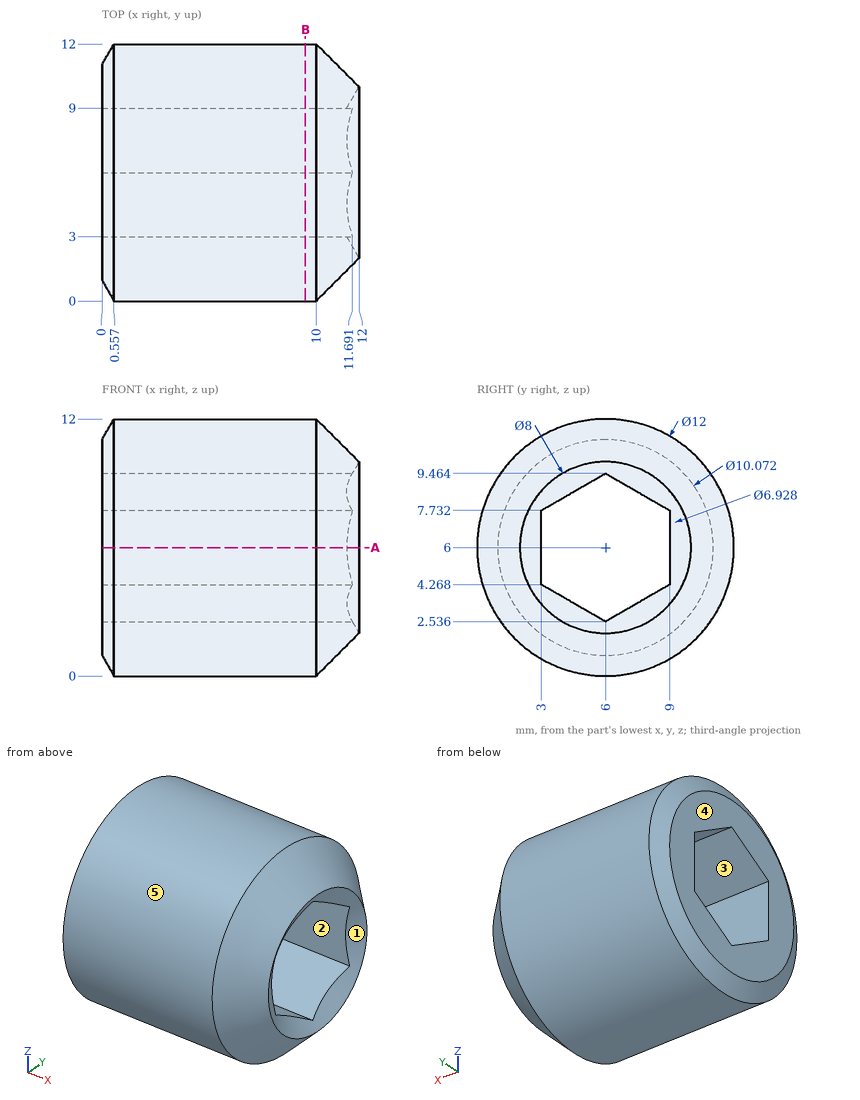
Can you work these out from the drawing? Everything is in mm from the part's minimum corner. A direction names the side the tool comes from. Coordinates: 2 decimals unless noted, no trailing zeros. Loops run counter-clockwise (first coordinate to the right, second up) from the corner with the lowest first, then second, coordinate; pieces in that order, holes last. Notation, with made-up numbers: (27.5, -2.75) - (85.5, -2.75) arc R13 cw to (85.5, 10.25) - close; hole circle Ø4 at (38.5, 39.5). An arc over 180 degrees is marked (long way). Put each result on its own line as item: value. Start each with the question number.
Item 1: If I drill on line 1 along Y through (x, z) = (1.75, 8.75) (1 decimal); line 2 along Z through (x, y) = (6.75, 3.5) (1 decimal); line 3 along Y through (x, z) = (1.5, 5) (1 decimal), over which ranges is the centre line in solid material (lowest first)?
Item 2: For pin 1 (1.5 mm diameter, centred on x = 3.5, y = 4.5, fed in from -Z); pin 2 (2 mm diameter, centred on x = 1.5, z = 9, fed in from -Y); pin 3 (1 mm diameter, centred on x = 10, z = 9.5, fed in from -Y) (1 decimal), each with a flat end and sliding along its axis, tell me the tip position at first contact or that it passes through.
Item 3: Suppose I cut it at B-B (x = 9.5). Please give me the cut outline in (y, z).
Item 4: Suppose I cut it at A-A (z = 6). Please give me the cut outline in (x, y).
Item 5: Which directions (+Z, -Z, +X, -X, +Y, -Y) give clear straight access to the entire face, cutting with the end or side of a thin tool? Please do the marked faces 1 and 2.
Item 6: If we mould it in two halves opening along Y, with no side actions, what happens to the marked faces 3, 4 and 5? For each: +Y half, -Y half, draft (parallel to the pull), parting line (faces both ways), or undercut.
Here are the results:
1. line 1: 0.7 to 4.8, 7.2 to 11.3
1. line 2: 0.5 to 4, 8 to 11.5
1. line 3: 0.1 to 3, 9 to 11.9
2. pin 1: z = 0.05
2. pin 2: y = 0.34
2. pin 3: y = 0.8
3. outline: circle Ø12 at (6, 6); hole (3, 4.27) - (6, 2.54) - (9, 4.27) - (9, 7.73) - (6, 9.46) - (3, 7.73) - close
4. outline: (0, 0.96) - (0.56, 0) - (10, 0) - (12, 2) - (11.42, 3) - (0, 3) - close; (0, 9) - (11.42, 9) - (12, 10) - (10, 12) - (0.56, 12) - (0, 11.04) - close
5. face 1: +X
5. face 2: +X, -X
6. face 3: undercut
6. face 4: draft
6. face 5: parting line
